Autodesk Inventor part; units mm, degrees
ref_plane "YZ Plane" through (0, 0, 0) normal (1, 0, 0) x (0, 1, 0)
ref_plane "XZ Plane" through (0, 0, 0) normal (0, 1, 0) x (-1, 0, 0)
ref_plane "XY Plane" through (0, 0, 0) normal (0, 0, 1) x (1, 0, 0)
sketch "Sketch1" plane through (0, 0, 0) normal (0, 0, 1) x (1, 0, 0)
  arc A0 (-20.5392, 17.1146) -> (-21.125, 15.7004) centre (-19.125, 15.7004) ccw
  line L0 (-21.125, -15.7004) -> (-21.125, 15.7004)
  arc A1 (-21.125, -15.7004) -> (-20.5392, -17.1146) centre (-19.125, -15.7004) ccw
  line L1 (-20.5392, -17.1146) -> (-17.1146, -20.5392)
  arc A2 (-17.1146, -20.5392) -> (-15.7004, -21.125) centre (-15.7004, -19.125) ccw
  line L2 (15.7004, -21.125) -> (-15.7004, -21.125)
  arc A3 (15.7004, -21.125) -> (17.1146, -20.5392) centre (15.7004, -19.125) ccw
  line L3 (20.5392, -17.1146) -> (17.1146, -20.5392)
  arc A4 (20.5392, -17.1146) -> (21.125, -15.7004) centre (19.125, -15.7004) ccw
  line L4 (21.125, 15.7004) -> (21.125, -15.7004)
  arc A5 (21.125, 15.7004) -> (20.5392, 17.1146) centre (19.125, 15.7004) ccw
  line L5 (20.5392, 17.1146) -> (17.1146, 20.5392)
  arc A6 (17.1146, 20.5392) -> (15.7004, 21.125) centre (15.7004, 19.125) ccw
  line L6 (-15.7004, 21.125) -> (15.7004, 21.125)
  arc A7 (-15.7004, 21.125) -> (-17.1146, 20.5392) centre (-15.7004, 19.125) ccw
  line L7 (-20.5392, 17.1146) -> (-17.1146, 20.5392)
  circle A8 centre (0, 0) radius 16
  circle A9 centre (-15.875, -15.875) radius 1.625
  circle A10 centre (15.875, 15.875) radius 1.625
  circle A11 centre (-15.875, 15.875) radius 1.625
  circle A12 centre (15.875, -15.875) radius 1.625
  circle A13 centre (0, 0) radius 12
  circle A14 centre (-15.875, 15.875) radius 2
  circle A15 centre (15.875, 15.875) radius 2
  circle A16 centre (15.875, -15.875) radius 2
  circle A17 centre (-15.875, -15.875) radius 2
  line L8 (-21.125, -15.7004) -> (-29.125, -15.7004)
  line L9 (-29.125, -15.7004) -> (-29.125, 21.125)
  line L10 (-29.125, 21.125) -> (-21.125, 21.125)
  line L11 (-21.125, 21.125) -> (-21.125, -15.7004)
  line L12 (15.7004, 21.125) -> (-29.125, 21.125)
  line L13 (-29.125, 21.125) -> (-29.125, 29.125)
  line L14 (-29.125, 29.125) -> (15.7004, 29.125)
  line L15 (15.7004, 29.125) -> (15.7004, 21.125)
  point P0 (0, 0)
  dimension "d0" = 24
  dimension "d1" = 4
  dimension "d2" = 4
  dimension "d3" = 4
  dimension "d4" = 4
  dimension "d77" = 8
  dimension "d78" = 8
extrude "Extrusion1" add sketch "Sketch1" along normal blind 5 contours L7 A7 L6 A6 L5 A5 L4 A4 L3 A3 L2 A2 L1 A1 L0 A0 | A8
sketch "Sketch3" plane through (0, 0, 5) normal (0, 0, 1) x (1, 0, 0)
  line L0 (-15.7004, 21.125) -> (15.7004, 21.125)
  line L1 (15.7004, 21.125) -> (-51.5519, 21.125)
  line L2 (-51.5519, 21.125) -> (-51.5519, 26.125)
  line L3 (-51.5519, 26.125) -> (15.7004, 26.125)
  line L4 (15.7004, 26.125) -> (15.7004, 21.125)
  line L5 (-21.125, 15.7004) -> (-21.125, -15.7004)
  line L6 (-21.125, -15.7004) -> (-26.125, -15.7004)
  line L7 (-26.125, -15.7004) -> (-26.125, 51.5519)
  line L8 (-26.125, 51.5519) -> (-21.125, 51.5519)
  line L9 (-21.125, 51.5519) -> (-21.125, -15.7004)
  arc A0 (-20.5392, 17.1146) -> (-21.125, 15.7004) centre (-19.125, 15.7004) ccw
  line L10 (15.7004, 21.125) -> (-15.7004, 21.125)
  line L11 (-21.125, 15.7004) -> (-15.7004, 21.125)
  line L12 (-15.7004, 21.125) -> (-26.1272, 31.5519)
  line L13 (-26.1272, 31.5519) -> (-31.5519, 26.1272)
  line L14 (-31.5519, 26.1272) -> (-21.125, 15.7004)
  line L15 (-31.5519, 26.1272) -> (-51.5519, 26.1272)
  line L16 (-51.5519, 26.1272) -> (-51.5519, 31.1272)
  line L17 (-51.5519, 31.1272) -> (-31.5519, 31.1272)
  line L18 (-31.5519, 31.1272) -> (-31.5519, 26.1272)
  line L19 (-26.1272, 31.5519) -> (-31.1272, 31.5519)
  line L20 (-31.1272, 31.5519) -> (-31.1272, 51.5519)
  line L21 (-31.1272, 51.5519) -> (-26.1272, 51.5519)
  line L22 (-26.1272, 51.5519) -> (-26.1272, 31.5519)
  line L23 (-31.5519, 31.1272) -> (-31.1272, 31.1272)
  line L24 (-31.1272, 31.1272) -> (-31.1272, 31.5519)
  point P0 (0, 0)
  point P1 (-31.5496, 26.125)
  point P2 (-26.125, 21.125)
  point P3 (-21.125, 21.125)
  point P4 (-21.125, 26.125)
  point P5 (-26.125, 31.5496)
  dimension "d11" = 5
  dimension "d12" = 5
  dimension "d79" = 5
  dimension "d80" = 5
  dimension "d81" = 20
  dimension "d82" = 20
  dimension "d83" = 0
  dimension "d84" = 0
extrude "Extrusion3" add sketch "Sketch3" against normal blind 40 contours L12 L3 L4 L0 | L1 L9 L3 L12 | L9 L14 L7 L1 | L1 L7 L3 L9 | L5 L6 L7 L14 | L1 L14 L3 L7 | L3 L7 L12 L9 | L12 L7 L8 L9 | L1 L2 L3 L14 | L3 L14 L13 L12 L7 | L13 L18 L23 L24 L19 | L19 L20 L21 L22 | L15 L16 L17 L18
sketch "Sketch4" plane through (0, 0, 5) normal (0, 0, 1) x (1, 0, 0)
  arc A0 (-15.7004, 21.125) -> (-17.1146, 20.5392) centre (-15.7004, 19.125) ccw
  line L0 (-17.1146, 20.5392) -> (-20.5392, 17.1146)
  arc A1 (-20.5392, 17.1146) -> (-21.125, 15.7004) centre (-19.125, 15.7004) ccw
  line L1 (-21.125, 26.125) -> (-21.125, 51.5519)
  line L2 (-51.5519, 21.125) -> (-26.125, 21.125)
  circle A2 centre (0, 0) radius 12
  circle A3 centre (-15.875, -15.875) radius 2
  circle A4 centre (15.875, -15.875) radius 2
  circle A5 centre (15.875, 15.875) radius 2
  circle A6 centre (-15.875, 15.875) radius 2
  line L3 (15.7004, 21.125) -> (15.7004, 26.125)
  line L4 (15.7004, 26.125) -> (-21.125, 26.125)
  line L5 (-21.125, 51.5519) -> (-26.125, 51.5519)
  line L6 (-26.125, 51.5519) -> (-26.125, 31.5496)
  line L7 (-31.5496, 26.125) -> (-51.5519, 26.125)
  line L8 (-51.5519, 26.125) -> (-51.5519, 21.125)
  line L9 (-26.125, 21.125) -> (-26.125, -15.7004)
  line L10 (-26.125, -15.7004) -> (-21.125, -15.7004)
  arc A7 (-21.125, -15.7004) -> (-20.5392, -17.1146) centre (-19.125, -15.7004) ccw
  line L11 (-20.5392, -17.1146) -> (-17.1146, -20.5392)
  arc A8 (-17.1146, -20.5392) -> (-15.7004, -21.125) centre (-15.7004, -19.125) ccw
  line L12 (-15.7004, -21.125) -> (15.7004, -21.125)
  arc A9 (15.7004, -21.125) -> (17.1146, -20.5392) centre (15.7004, -19.125) ccw
  line L13 (17.1146, -20.5392) -> (20.5392, -17.1146)
  arc A10 (20.5392, -17.1146) -> (21.125, -15.7004) centre (19.125, -15.7004) ccw
  line L14 (21.125, -15.7004) -> (21.125, 15.7004)
  arc A11 (21.125, 15.7004) -> (20.5392, 17.1146) centre (19.125, 15.7004) ccw
  line L15 (20.5392, 17.1146) -> (17.1146, 20.5392)
  arc A12 (17.1146, 20.5392) -> (15.7004, 21.125) centre (15.7004, 19.125) ccw
  line L16 (-26.125, 31.5496) -> (-26.1272, 31.5519)
  line L17 (-26.1272, 31.5519) -> (-26.1272, 51.5519)
  line L18 (-26.1272, 51.5519) -> (-31.1272, 51.5519)
  line L19 (-31.1272, 51.5519) -> (-31.1272, 31.1272)
  line L20 (-31.1272, 31.1272) -> (-51.5519, 31.1272)
  line L21 (-51.5519, 31.1272) -> (-51.5519, 26.1272)
  line L22 (-51.5519, 26.1272) -> (-31.5519, 26.1272)
  line L23 (-31.5519, 26.1272) -> (-31.5496, 26.125)
  line L24 (-21.125, 15.7004) -> (-21.125, 21.125)
  line L25 (-21.125, 21.125) -> (-15.7004, 21.125)
  point P0 (0, 0)
extrude "Extrusion4" add sketch "Sketch4" against normal blind 5 contours A0 L0 A1 L24 L25
sketch "Sketch11" plane through (0, 0, 5) normal (0, 0, 1) x (1, 0, 0)
  line L0 (-26.125, 21.125) -> (-26.125, 51.5519)
  line L1 (-26.125, 26.125) -> (-19.1264, 26.125)
  line L2 (-19.1264, 26.125) -> (-19.1264, 59.1574)
  line L3 (-19.1264, 59.1574) -> (-26.125, 59.1574)
  line L4 (-26.125, 59.1574) -> (-26.125, 26.125)
  line L5 (-51.5519, 26.125) -> (-51.5519, 21.125)
  line L6 (-51.5519, 26.125) -> (-26.125, 26.125)
  line L7 (-26.125, 26.125) -> (-26.125, 13.3287)
  line L8 (-26.125, 13.3287) -> (-51.5519, 13.3287)
  line L9 (-51.5519, 13.3287) -> (-51.5519, 26.125)
  line L10 (-26.125, 26.125) -> (-55.9242, 26.125)
  line L11 (-55.9242, 26.125) -> (-55.9242, 63.8305)
  line L12 (-55.9242, 63.8305) -> (-26.125, 63.8305)
  line L13 (-26.125, 63.8305) -> (-26.125, 26.125)
  point P0 (0, 0)
  point P1 (-26.125, 46.125)
extrude "Extrusion9" cut sketch "Sketch11" against normal blind 20
sketch "Sketch7" plane through (0, 0, -35) normal (0, 0, -1) x (-1, 0, 0)
  line L0 (21.625, 21.625) -> (-23.2924, 21.625)
  line L1 (-23.2924, 21.625) -> (-23.2924, -21.9013)
  line L2 (-23.2924, -21.9013) -> (21.625, -21.9013)
  line L3 (21.625, -21.9013) -> (21.625, 21.625)
  line L4 (-15.7004, 21.125) -> (51.5519, 21.125)
  line L5 (21.125, 51.5519) -> (21.125, -15.7004)
  point P0 (0, 0)
  point P1 (21.125, 21.125)
  dimension "d35" = 0.5
  dimension "d36" = 0.5
extrude "Extrusion7" cut sketch "Sketch7" against normal blind 35
sketch "Sketch12" plane through (0, 0, -35) normal (0, 0, -1) x (-1, 0, 0)
  line L0 (51.5519, 21.125) -> (51.5519, 26.125)
  line L1 (-15.7004, 26.125) -> (26.125, 26.125)
  line L2 (51.5519, 21.125) -> (27.0552, 21.125)
  line L3 (27.0552, 21.125) -> (27.0552, 26.125)
  line L4 (27.0552, 26.125) -> (51.5519, 26.125)
  line L5 (51.5519, 26.125) -> (51.5519, 21.125)
  line L6 (26.125, 51.5519) -> (21.125, 51.5519)
  line L7 (-15.7004, 21.625) -> (21.625, 21.625)
  line L8 (26.125, 51.5519) -> (21.125, 51.5519)
  line L9 (21.125, 51.5519) -> (21.125, 21.625)
  line L10 (21.125, 21.625) -> (26.125, 21.625)
  line L11 (26.125, 21.625) -> (26.125, 51.5519)
  line L12 (51.5519, 26.125) -> (31.5496, 26.125)
  line L13 (21.125, 51.5519) -> (21.125, 26.125)
  line L14 (26.125, 51.5519) -> (21.125, 51.5519)
  line L15 (26.125, 31.5496) -> (26.125, 51.5519)
  line L16 (26.1272, 31.5519) -> (26.125, 31.5496)
  line L17 (26.1272, 51.5519) -> (26.1272, 31.5519)
  line L18 (31.1272, 51.5519) -> (26.1272, 51.5519)
  line L19 (31.1272, 31.1272) -> (31.1272, 51.5519)
  line L20 (51.5519, 31.1272) -> (31.1272, 31.1272)
  line L21 (51.5519, 26.1272) -> (51.5519, 31.1272)
  line L22 (31.5519, 26.1272) -> (51.5519, 26.1272)
  line L23 (31.5496, 26.125) -> (31.5519, 26.1272)
  line L24 (51.5519, 26.125) -> (31.5496, 26.125)
  line L25 (51.5519, 21.125) -> (51.5519, 26.125)
  line L26 (26.125, 21.125) -> (51.5519, 21.125)
  line L27 (26.125, 26.125) -> (26.125, 21.125)
  line L28 (21.125, 26.125) -> (26.125, 26.125)
  point P0 (0, 0)
  point P1 (51.5519, 26.125)
  point P2 (26.125, 26.125)
  point P3 (21.125, 51.5519)
  point P4 (21.125, 26.125)
  dimension "d54" = 5
  dimension "d55" = 5
  dimension "d56" = 4.5
  dimension "d57" = 0.5
extrude "Extrusion10" add sketch "Sketch12" along normal blind 20
sketch "Sketch13" plane through (-51.5519, 21.125, -15) normal (0, -1, 0) x (1, 0, 0)
  circle A0 centre (10, -30) radius 2.5
  circle A1 centre (10, -10) radius 2.5
  line L0 (24.4966, -40) -> (0, -40)
  line L1 (0, 0) -> (0, -40)
  point P0 (51.5519, 15)
  point P1 (0, -20)
  dimension "d60" = 10
  dimension "d61" = 10
  dimension "d62" = 5
  dimension "d63" = 5
  dimension "d64" = 20
  dimension "d65" = 10
extrude "Extrusion11" cut sketch "Sketch13" against normal blind 20
sketch "Sketch14" plane through (-21.125, 26.125, -15) normal (-1, 0, 0) x (0, 0, 1)
  circle A0 centre (-10, 15.4269) radius 2.5
  circle A1 centre (-30, 15.4269) radius 2.5
  line L0 (0, 5.4246) -> (0, 25.4269)
  line L1 (0, 25.4269) -> (-40, 25.4269)
  point P0 (15, -26.125)
  point P1 (0, 0)
  point P2 (20, 25.4269)
  point P3 (-20, 25.4269)
  dimension "d68" = 10
  dimension "d69" = 10
  dimension "d70" = 20
  dimension "d71" = 10
  dimension "d72" = 5
  dimension "d73" = 5
extrude "Extrusion12" cut sketch "Sketch14" along normal mid plane 40
fillet "Fillet1" radius 5 2 edges at (-21.125, 26.125, -25) (-26.125, 21.125, -25)
sketch "Sketch15" plane through (0, 0, -35) normal (0, 0, -1) x (-1, 0, 0)
  line L0 (21.125, 21.625) -> (21.125, 31.125)
  arc A0 (16.125, 26.125) -> (21.125, 31.125) centre (16.125, 31.125) ccw
  line L1 (16.125, 26.125) -> (-15.7004, 26.125)
  line L2 (-15.7004, 26.125) -> (-15.7004, 21.625)
  line L3 (-15.7004, 21.625) -> (21.125, 21.625)
  line L4 (26.125, 21.125) -> (26.125, 21.625)
  line L5 (26.125, 21.625) -> (21.625, 21.625)
  line L6 (21.625, 21.625) -> (21.625, -15.7004)
  line L7 (21.625, -15.7004) -> (26.125, -15.7004)
  line L8 (26.125, -15.7004) -> (26.125, 16.125)
  arc A1 (31.125, 21.125) -> (26.125, 16.125) centre (31.125, 16.125) ccw
  line L9 (26.125, 21.125) -> (31.125, 21.125)
  point P0 (0, 0)
extrude "Extrusion13" add sketch "Sketch15" along normal blind 20
equation "\"d36\" = d35"
properties part number "StepperXYHolder"
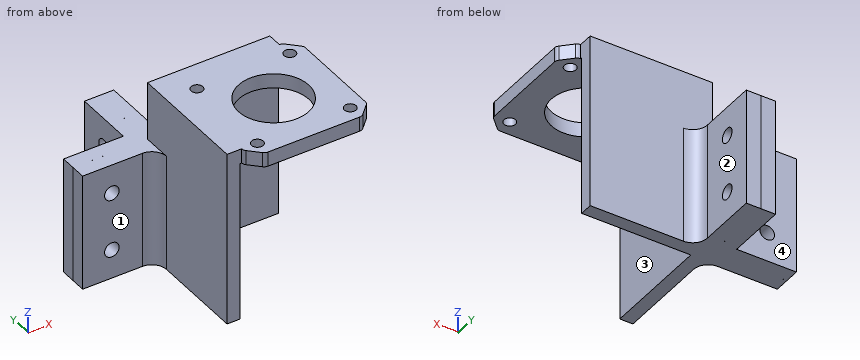
Could you check a few things on this model? Use its own coordinates, in mm. Face numbers are marked on the shaded views. A direction names the side the tool comes from. Give positions to 0.01 mm unless a question says otherwise; leave off trailing zeros. Write each loop counter-clockwise with the first axis right and the second up, starting at its lowest first coordinate (ties: lowest second). Pieces come first, ordered by that corner, then holes. Notation, with made-up numbers: (27.5, 63) -> (78.5, 63) arc R33 cw to (78.5, 100) -> close; hole circle Ø9 at (77.5, -1.5). An arc over 180 degrees is marked (long way). Answer as a JSON object with one key per item and string values.
Q1. Please list where these lines run through material, in increasing order: L1, parallel to Y at x = -24.9, z = -45; L2, parallel to X at y = -3, z = -11.5 (3 decimals); L3, parallel to Z at x = -39.5, y = 30.
Taken from the geometry:
{"L1": "y = -15.7 to 39.05, 44.05 to 51.55", "L2": "x = -26.125 to -21.625", "L3": "z = -55 to -46.43, -43.57 to -26.43, -23.57 to -15"}
Q2. Suppose I cut it at A-A on x = -37. Write out the boundary of the cut face in (y, z) (3 decimals).
Taken from the geometry:
{"outline": "(21.125, -55) -> (26.125, -55) -> (26.125, -15) -> (21.125, -15) -> close; (26.127, -55) -> (31.127, -55) -> (31.127, -15) -> (26.127, -15) -> close"}
Q3. Suppose I cut it at B-B on y = 0. Write out the boundary of the cut face in (x, z) (3 decimals).
Taken from the geometry:
{"outline": "(-26.125, -55) -> (-21.625, -55) -> (-21.625, 0) -> (-12, 0) -> (-12, 5) -> (-26.125, 5) -> close; (12, 0) -> (21.125, 0) -> (21.125, 5) -> (12, 5) -> close"}
Q4. Suppose I cut it at D-D on z = -25. Count the separate pieces of the cut face and the enclosed holes in it, then the cut area to 3 significant figures.
Taken from the geometry:
{"separate pieces": "5", "enclosed holes": "0", "area": "750 mm²"}
Q5. Which directions (+Z, -Z, +X, -X, +Y, -Y) give clear straight access to the entire face, cutting with the end or side of a thin tool? Please do the marked faces 1, 2, 3 and 4.
Taken from the geometry:
{"face 1": "+Z, -Z, -X, -Y", "face 2": "+Z, -Z, +X, +Y", "face 3": "-Z, +X, -Y", "face 4": "+Z, -Z, -X, +Y"}
Q6. Will these pins go through, and if not, where does the flat tip stop? pin 1 Ø6 at (x, z) = (-38, -34) entering from +Y; pin 2 Ø6 at (y, z) = (41.5, -40) entering from +X (3 decimals); pin 3 Ø3 at (y, z) = (41.55, -45) entering from -X; pin 4 Ø18.5 at (x, z) = (-2, -28.5) entering from -Y (3 decimals).
Taken from the geometry:
{"pin 1": "stops at y = 31.13", "pin 2": "stops at x = -21.125", "pin 3": "passes through", "pin 4": "stops at y = 21.625"}
